Could you check a few things on this model? Use its own coordinates, in mm. Face numbers are marked on the shaded views. A direction names the side the tool comes from. Round coordinates to 2 decimals unless told otherwise and drop trailing zeros. Order: outer loops, then holes, each group sorted by start corner. A loop starts at its lowest first (then second) coordinate and runs counter-clockwise, first axis right, second up. Notation, with made-up numbers: (70.5, 8.5) -> (77.5, 8.5) arc R32 ccw to (77.5, 34.5) -> close; hole circle Ø10 at (-30, 44). An arc over 180 degrees is marked (long way). Put each result on its own line as item: value. Start each with the question number.
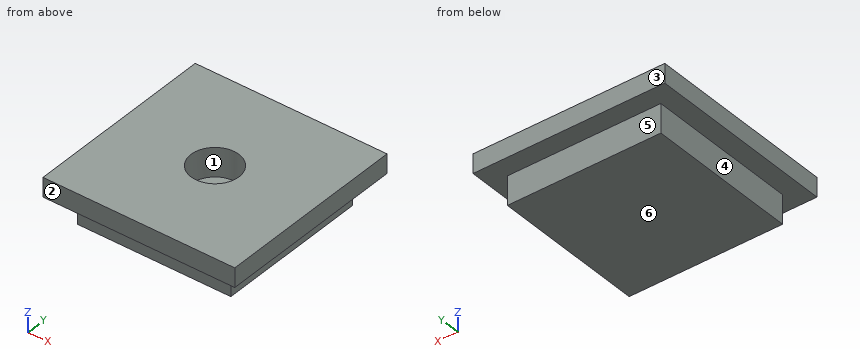
from build123d import *

# Parameters (mm, degrees)
F0_W     = 25.4
F0_H     = 25.4
F1_DEPTH = 2.54
F2_W     = 20.32
F2_H     = 20.32
F3_DEPTH = 3.81
F4_R     = 3.175
F5_DEPTH = 3.81


with BuildPart() as f1:
    # F0 (on Top) → F1 (new body)
    with BuildSketch(Plane.XY):
        Rectangle(F0_W, F0_H)
    extrude(amount=F1_DEPTH)

    # F2 (on face) → F3 (join)
    with BuildSketch(Plane(origin=(0, 0, 0), x_dir=(1, 0, 0), z_dir=(0, 0, -1))):
        Rectangle(F2_W, F2_H)
    extrude(amount=F3_DEPTH)

    # F4 (on face) → F5 (cut)
    with BuildSketch(Plane.XY.offset(2.54)):
        Circle(F4_R)
    extrude(amount=-F5_DEPTH, mode=Mode.SUBTRACT)


solid = f1.part
1. For pin 1 Ø5 at (x, y) = (0, -0.5) entering from +Z; pin 2 Ø1.1 at (y, z) = (3.5, -1.5) entering from -X; pin 3 Ø3 at (y, z) = (-2.5, -0.5) entering from +X; pin 4 Ø1.1 at (x, z) = (-2.5, -1.5) entering from +Y, each with a flat end and sliding along its axis, tell me the tip position at first contact or that it passes through.
2. If we section it at D-D, the plane y = -6: Please give me the cut outline in (x, z).
3. I need wall thicknesses on L1, parallel to Y at x = 0, z = 1.45 (3 decimals); L2, parallel to X at y = -4.5, z = -2.5; L3, parallel to Z at x = 0, y = -2.5. Which ranges of each line are inside material? Lowest first, please.
4. Thinking about a two-plate mould opening in Y: for the marked faces 1, 2, 3 and 4, which applies, +Y half, -Y half, draft (parallel to the pull), parting line (faces both ways), or undercut?
5. If we section it at A-A, the plane x = 0: Please give me the cut outline in (y, z) (3 decimals), then the cut area to 3 significant figures.
6. Which directions (+Z, -Z, +X, -X, +Y, -Y) give clear straight access to the entire face, cutting with the end or side of a thin tool? Please do the marked faces 5 and 6.
7. If we section it at C-C, the plane z = -0.5: Please give me the cut outline in (x, y) (3 decimals), then the cut area to 3 significant figures.
Results below:
1. pin 1: z = -1.27
1. pin 2: x = -10.16
1. pin 3: x = 12.7
1. pin 4: y = 10.16
2. outline: (-12.7, 0) -> (-10.16, 0) -> (-10.16, -3.81) -> (10.16, -3.81) -> (10.16, 0) -> (12.7, 0) -> (12.7, 2.54) -> (-12.7, 2.54) -> close
3. L1: -12.7 to -3.175, 3.175 to 12.7
3. L2: -10.16 to 10.16
3. L3: -3.81 to -1.27
4. face 1: undercut
4. face 2: -Y half
4. face 3: +Y half
4. face 4: draft
5. outline: (-12.7, 0) -> (-10.16, 0) -> (-10.16, -3.81) -> (10.16, -3.81) -> (10.16, 0) -> (12.7, 0) -> (12.7, 2.54) -> (3.175, 2.54) -> (3.175, -1.27) -> (-3.175, -1.27) -> (-3.175, 2.54) -> (-12.7, 2.54) -> close
5. area: 118 mm2
6. face 5: -Z, +X, -X, +Y
6. face 6: -Z, +X, -X, +Y, -Y
7. outline: (-10.16, -10.16) -> (10.16, -10.16) -> (10.16, 10.16) -> (-10.16, 10.16) -> close; hole circle Ø6.35 at (0, 0)
7. area: 381 mm2
